from build123d import *

# Parameters (mm, degrees)
F1_DEPTH = 15
F3_DEPTH = 100
F5_DEPTH = 12.5


with BuildPart() as f1:
    # F0 (on Front) → F1 (new body, symmetric)
    with BuildSketch(Plane.XZ):
        with BuildLine():
            ThreePointArc((37.317329624, 30.4986087275), (24.902598062, 33.210330732), (12.2824249303, 34.6970136545))
            ThreePointArc((12.2824249303, 34.6970136545), (0, 35.1170361544), (-12.2824249303, 34.6970136545))
            ThreePointArc((-12.2824249303, 34.6970136545), (-24.902598062, 33.210330732), (-37.317329624, 30.4986087275))
            Line((-37.317329624, 30.4986087275), (-65, 23.01738))
            Line((-65, 23.01738), (-62.3910963169, 13.3636956478))
            Line((-62.3910963169, 13.3636956478), (-34.7084259409, 20.8449243753))
            ThreePointArc((-34.7084259409, 20.8449243753), (-23.2486737298, 23.3480523794), (-11.5992831467, 24.7203750772))
            ThreePointArc((-11.5992831467, 24.7203750772), (0, 25.1170361544), (11.5992831467, 24.7203750772))
            ThreePointArc((11.5992831467, 24.7203750772), (23.2486737298, 23.3480523794), (34.7084259409, 20.8449243753))
            Line((34.7084259409, 20.8449243753), (62.3910963169, 13.3636956478))
            Line((62.3910963169, 13.3636956478), (65, 23.01738))
            Line((65, 23.01738), (37.317329624, 30.4986087275))
        make_face()
    extrude(amount=F1_DEPTH, both=True)

    # F2 (on Right) → F3 (cut, symmetric)
    with BuildSketch(Plane.YZ):
        Polygon((-1.875644347, 7), (-17, 63.4448637287), (-17, 0), (0, 0), (17, 0), (17, 63.4448637287), (1.875644347, 7), align=None)
    extrude(amount=F3_DEPTH, both=True, mode=Mode.SUBTRACT)

    # F4 (on Front) → F5 (cut, symmetric)
    with BuildSketch(Plane.XZ):
        with BuildLine():
            ThreePointArc((11.7359115034, 26.7157027926), (0, 27.1170361544), (-11.7359115034, 26.7157027926))
            ThreePointArc((-11.7359115034, 26.7157027926), (-23.5794585962, 25.32050805), (-35.2302066775, 22.7756612458))
            ThreePointArc((-35.2302066775, 22.7756612458), (-37.021132821, 21.7365411239), (-38.0525602966, 19.9411736291))
            Line((-38.0525602966, 19.9411736291), (-34.7084259409, 20.8449243753))
            ThreePointArc((-34.7084259409, 20.8449243753), (-23.2486737298, 23.3480523794), (-11.5992831467, 24.7203750772))
            ThreePointArc((-11.5992831467, 24.7203750772), (0, 25.1170361544), (11.5992831467, 24.7203750772))
            ThreePointArc((11.5992831467, 24.7203750772), (23.2486737298, 23.3480523794), (34.7084259409, 20.8449243753))
            Line((34.7084259409, 20.8449243753), (38.0525602966, 19.9411736291))
            ThreePointArc((38.0525602966, 19.9411736291), (37.021132821, 21.7365411239), (35.2302066775, 22.7756612458))
            ThreePointArc((35.2302066775, 22.7756612458), (23.5794585962, 25.32050805), (11.7359115034, 26.7157027927))
        make_face()
    extrude(amount=F5_DEPTH, both=True, mode=Mode.SUBTRACT)


solid = f1.part
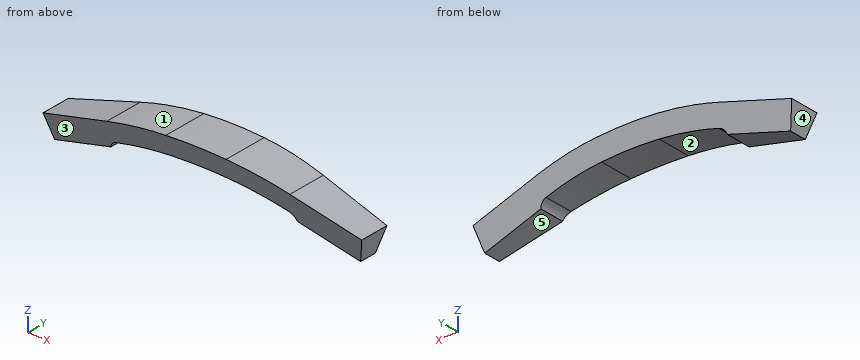
Design review of the part built by this model. Coordinates are the model's own, in mm. Face numbers are marked on the shaded views. A direction names the side the tool comes from. Coordinates: 2 decimals unless noted, no trailing zeros. Order: outer loops, then holes, each group sorted by start corner. A loop starts at its lowest first (then second) coordinate and runs counter-clockwise, first axis right, second up.
Item 1: Take a section at C-C, the plane z = 25. Write out the cut boundary in (x, y), then the cut area to 3 significant figures.
Item 2: For line 1 (Z direction, x = 2.5, y = -0.5); line 2 (X direction, y = 5, z = 22.25); line 3 (X direction, y = 2, z = 20), list the stretches that pass through material, from the lowest coordinate up.
Item 3: Take a section at A-A, the plane z = 14.75. Write out the cut boundary in (x, y).
Item 4: Take a section at D-D, the plane x = -26. Write out the cut boundary in (y, z).
Item 5: For the marked faces 1 and 2, list the 3-axis set-ups (+Z, -Z, +X, -X, +Y, -Y) from which the entire face can be reached by the end or side of a thin tool; tool diameter is ignored.
Item 6: For pin 1 Ø4 at (x, y) = (-17.5, -2.5) entering from -Z; pin 2 Ø8 at (x, z) = (21, 19.5) entering from +Y; pin 3 Ø10 at (y, z) = (1, 19) entering from +X; pin 4 Ø2 at (x, y) = (22, 3.5) entering from -Z, all flat-tipped, find the tip position at first contact; note any pin that passes through.
Item 7: The part is to be moulded in two halves that separate along X. For the marked faces 3, 4 and 5, say which applies: pulls with the +X half, pulls with the -X half, needs draft (parallel to the pull), parting line crosses it, or undercut.
Item 8: Take a section at B-B, the plane y = -2.5. Write out the cut boundary in (x, z).
The answers:
1. outline: (-57.66, -6.7) - (-25.41, -6.7) - (-25.41, 6.7) - (-57.66, 6.7) - close; (25.41, -6.7) - (57.66, -6.7) - (57.66, 6.7) - (25.41, 6.7) - close
1. area: 864 mm2
2. line 1: z = 27.1 to 35.1
2. line 2: x = -64.79 to -36.39, 36.39 to 64.79
2. line 3: x = -64.18 to -38.04, 38.04 to 64.18
3. outline: (-62.77, -3.95) - (-57.26, -3.95) - (-57.26, 3.95) - (-62.77, 3.95) - close; (57.26, -3.95) - (62.77, -3.95) - (62.77, 3.95) - (57.26, 3.95) - close
4. outline: (-8.85, 33.02) - (-6.67, 24.89) - (6.67, 24.89) - (8.85, 33.02) - close
5. face 1: +Z, -X, +Y, -Y
5. face 2: -Z, +Y, -Y
6. pin 1: stops at z = 25.93
6. pin 2: passes through
6. pin 3: stops at x = 65
6. pin 4: stops at z = 25.42
7. face 3: needs draft
7. face 4: pulls with the -X half
7. face 5: undercut
8. outline: (-65, 23.02) - (-62.39, 13.36) - (-38.05, 19.94) arc R4 cw to (-35.23, 22.78) arc R122 cw to (-11.74, 26.72) arc R171.79 cw to (11.74, 26.72) arc R122 cw to (35.23, 22.78) arc R4 cw to (38.05, 19.94) - (62.39, 13.36) - (65, 23.02) - (37.32, 30.5) arc R130 ccw to (12.28, 34.7) arc R179.79 ccw to (-12.28, 34.7) arc R130 ccw to (-37.32, 30.5) - close
